Autodesk Fusion 360 part; units mm, degrees
sketch "Sketch1" plane through (0, 0, 0) normal (0, 1, 0) x (1, 0, 0)
  line L0 (-2.8868, 5) -> (-5.7735, 0)
  line L1 (-5.7735, 0) -> (-2.8868, -5)
  line L2 (-2.8868, -5) -> (2.8868, -5)
  line L3 (2.8868, -5) -> (5.7735, 0)
  line L4 (5.7735, 0) -> (2.8868, 5)
  line L5 (2.8868, 5) -> (-2.8868, 5)
  circle A0 centre (0, 0) radius 7
  dimension "d1" = 5
  dimension "d2" = 14
extrude "Extrude1" add sketch "Sketch1" along normal blind 10
sketch "Sketch2" plane through (-4.3301, 0, -2.5) normal (0.866, 0, 0.5) x (0.5, 0, -0.866)
  line L0 (-2.8868, 0) -> (2.8868, 0)
  line L1 (2.8868, 0) -> (2.8868, 10)
  line L2 (2.8868, 10) -> (-2.8868, 10)
  line L3 (-2.8868, 10) -> (-2.8868, 0)
  circle A0 centre (0, 5) radius 1.5
  dimension "d5" = 3
  dimension "d6" = 5
extrude "Extrude2" cut sketch "Sketch2" against normal through all contours A0
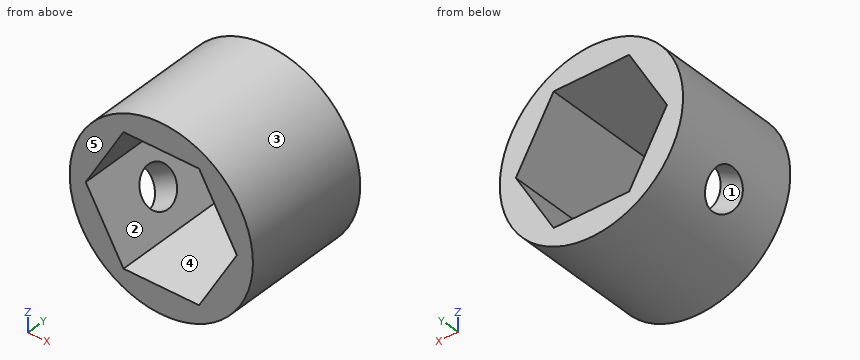
The model under review builds one solid part; all positions refer to its coordinate system, in mm. Face numbers are marked on the shaded views. A direction names the side the tool comes from. Round coordinates to 2 decimals unless told otherwise and drop trailing zeros. Order: outer loops, then holes, each group sorted by start corner. A loop starts at its lowest first (then second) coordinate and runs counter-clockwise, first axis right, second up. Notation, with made-up numbers: (-30, -30) - (1, -30) arc R17 ccw to (1, -9) - close; hole circle Ø4 at (-1, 48.25). An arc over 180 degrees is marked (long way). Answer in a Markdown table with one row per item.
(1) Take a section at A-A on x = 0. Write out the cut boundary in (y, z), plus the area to 3 significant figures.
Result set:
| item | result |
|---|---|
| outline | (0, -7) - (10, -7) - (10, -5) - (0, -5) - close; (0, 5) - (10, 5) - (10, 7) - (0, 7) - close |
| area | 40.0 mm2 |
(2) For line 1 (Z direction, x = -0.5, y = 7.75); line 2 (X direction, y = 9.5, z = -1.5); line 3 (Z direction, x = -3.25, y = 6.5), list the stretches that pass through material, from the lowest coordinate up. Write a range as from..to.
Result set:
| item | result |
|---|---|
| line 1 | z = -6.98..-5, 5..6.98 |
| line 2 | x = -6.84..-4.91, 4.91..6.84 |
| line 3 | z = -6.2..-4.37, 4.37..6.2 |
(3) Clearance check with flat-ended pins moving along their axes: P1, Ø1, axis at x = 3, y = 6.5, coming from the -Z side; P2, Ø1.5, axis at x = -3, y = 5.5, coming from the +Z side; P3, Ø4, axis at x = -5, y = 4, coming from the -Z side. State where each tip first meets the part, or that it passes through.
Result set:
| item | result |
|---|---|
| P1 | stops at z = -6.54 |
| P2 | stops at z = 6.63 |
| P3 | stops at z = -6.32 |
(4) Take a section at D-D on x = 5.5. Write out the cut boundary in (y, z).
Result set:
| item | result |
|---|---|
| outline | (0, -4.33) - (10, -4.33) - (10, -0.47) - (0, -0.47) - close; (0, 0.47) - (10, 0.47) - (10, 4.33) - (0, 4.33) - close |
(5) Machinability: for the marked faces 1 and 2, which of the approach directions +Z, -Z, +X, -X, +Y, -Y give a long, thin tool a straight path to every point of the face, cutting with its end or side? Answer none if there is none.
Result set:
| item | result |
|---|---|
| face 1 | none |
| face 2 | +Y, -Y |
(6) Mouldability with a two-part tool opening along X and no side actions: class the marked faces 3, 4 and 5 as released by +X, released by -X, zero draft, split by the parting line, or undercut.
Result set:
| item | result |
|---|---|
| face 3 | split by the parting line |
| face 4 | undercut |
| face 5 | zero draft |
(7) Take a section at B-B on y = 7.75. Write out the cut boundary in (x, z), plus the area to 3 significant figures.
Result set:
| item | result |
|---|---|
| outline | circle Ø14 at (0, 0); hole (-5.77, 0) - (-2.89, -5) - (2.89, -5) - (5.77, 0) - (2.89, 5) - (-2.89, 5) - close |
| area | 67.3 mm2 |
(8) Take a section at C-C on y = 4.5. Write out the cut boundary in (x, z).
Result set:
| item | result |
|---|---|
| outline | (-6.64, -2.2) - (-5.04, -1.28) - (-5.77, 0) - (-2.89, 5) - (2.89, 5) - (5.77, 0) - (2.89, -5) - (-2.89, -5) - (-3.62, -3.72) - (-5.23, -4.65) arc R7 ccw (long way) to start |
